Input: part model. Units: mm. Frame: model coordinates. Face numbers are marked on the shaded views. Coordinates: 2 decimals unless noted, no trailing zeros. Write each loop counter-clockwise with the first axis right and the second up, starting at its lowest first coordinate (ties: lowest second). Pieces come first, ordered by that corner, then holes. Notation, with made-up numbers: M 56,62 L 92,62 A31 cw 92,92 Z; hole C 26,50.5 d11. An arc over 180 degrees is marked long. Use CSV: the item, a comma, the result in double quotes.
```python
from build123d import *

# Parameters (mm, degrees)
SKETCH1_R           = 5.1
BOSS_EXTRUDE1_DEPTH = 4
BOSS_EXTRUDE2_START = -4
BOSS_EXTRUDE2_DEPTH = 4
SKETCH3_R           = 2.5
BOSS_EXTRUDE3_DEPTH = 4
SKETCH4_R           = 1.15
CUT_EXTRUDE1_DEPTH  = 4
FILLET1_R           = 10
FILLET2_R           = 1.5
FILLET3_R           = 5
SKETCH5_W           = 20.86
SKETCH5_H           = 29
BOSS_EXTRUDE4_DEPTH = 4
SKETCH6_W           = 4
SKETCH6_H           = 29
BOSS_EXTRUDE5_DEPTH = 12
FILLET4_R           = 10
FILLET5_R           = 2


with BuildPart() as part:
    # Sketch1 → Boss-Extrude1 (new body)
    with BuildSketch(Plane(origin=(0, 0, 0), x_dir=(1, 0, 0), z_dir=(0, 1, 0))):
        with BuildLine():
            ThreePointArc((-42.589636172, 29.834927363), (-52, 0), (-42.589636172, -29.834927363))
            ThreePointArc((-42.589636172, -29.834927363), (-41.790010768, -41.790010768), (-29.834927363, -42.589636172))
            ThreePointArc((-29.834927363, -42.589636172), (0, -52), (29.834927363, -42.589636172))
            ThreePointArc((29.834927363, -42.589636172), (41.790010768, -41.790010768), (42.589636172, -29.834927363))
            ThreePointArc((42.589636172, -29.834927363), (52, 0), (42.589636172, 29.834927363))
            ThreePointArc((42.589636172, 29.834927363), (41.790010768, 41.790010768), (29.834927363, 42.589636172))
            ThreePointArc((29.834927363, 42.589636172), (0, 52), (-29.834927363, 42.589636172))
            ThreePointArc((-29.834927363, 42.589636172), (-41.790010768, 41.790010768), (-42.589636172, 29.834927363))
        make_face()
        with Locations(Location((-35.355339059, -35.355339059, 0), (0, 0, 270))):
            Circle(SKETCH1_R, mode=Mode.SUBTRACT)
        with Locations(Location((35.355339059, -35.355339059, 0), (0, 0, 270))):
            Circle(SKETCH1_R, mode=Mode.SUBTRACT)
        with BuildLine():
            ThreePointArc((-27.258640426, -39.509068859), (-28.920667351, -28.920667351), (-39.509068859, -27.258640426))
            ThreePointArc((-39.509068859, -27.258640426), (-48, 0), (-39.509068859, 27.258640426))
            ThreePointArc((-39.509068859, 27.258640426), (-28.920667351, 28.920667351), (-27.258640426, 39.509068859))
            ThreePointArc((-27.258640426, 39.509068859), (0, 48), (27.258640426, 39.509068859))
            ThreePointArc((27.258640426, 39.509068859), (28.920667351, 28.920667351), (39.509068859, 27.258640426))
            ThreePointArc((39.509068859, 27.258640426), (48, 0), (39.509068859, -27.258640426))
            ThreePointArc((39.509068859, -27.258640426), (28.920667351, -28.920667351), (27.258640426, -39.509068859))
            ThreePointArc((27.258640426, -39.509068859), (0, -48), (-27.258640426, -39.509068859))
        make_face(mode=Mode.SUBTRACT)
        with Locations(Location((-35.355339059, 35.355339059, 0), (0, 0, 270))):
            Circle(SKETCH1_R, mode=Mode.SUBTRACT)
        with Locations(Location((35.355339059, 35.355339059, 0), (0, 0, 270))):
            Circle(SKETCH1_R, mode=Mode.SUBTRACT)
    extrude(amount=BOSS_EXTRUDE1_DEPTH)

    # Sketch2 → Boss-Extrude2 (add)
    with BuildSketch(Plane(origin=(0, 4, 0), x_dir=(1, 0, 0), z_dir=(0, 1, 0)).offset(BOSS_EXTRUDE2_START)):
        with BuildLine():
            ThreePointArc((-26.255339059, 35.355339059), (-26.311135203, 34.349169788), (-26.477839411, 33.355339059))
            Line((-26.477839411, 33.355339059), (26.477839411, 33.355339059))
            ThreePointArc((26.477839411, 33.355339059), (26.255339059, 35.355339059), (26.477839411, 37.355339059))
            Line((26.477839411, 37.355339059), (-26.477839411, 37.355339059))
            ThreePointArc((-26.477839411, 37.355339059), (-26.311135203, 36.36150833), (-26.255339059, 35.355339059))
        make_face()
        with BuildLine():
            Line((-33.355339059, -26.477839411), (-33.355339059, 26.477839411))
            ThreePointArc((-33.355339059, 26.477839411), (-35.355339059, 26.255339059), (-37.355339059, 26.477839411))
            Line((-37.355339059, 26.477839411), (-37.355339059, -26.477839411))
            ThreePointArc((-37.355339059, -26.477839411), (-35.355339059, -26.255339059), (-33.355339059, -26.477839411))
        make_face()
        with BuildLine():
            ThreePointArc((37.355339059, 26.477839411), (35.355339059, 26.255339059), (33.355339059, 26.477839411))
            Line((33.355339059, 26.477839411), (33.355339059, -26.477839411))
            ThreePointArc((33.355339059, -26.477839411), (35.355339059, -26.255339059), (37.355339059, -26.477839411))
            Line((37.355339059, -26.477839411), (37.355339059, 26.477839411))
        make_face()
        with BuildLine():
            Line((26.477839411, -33.355339059), (-26.477839411, -33.355339059))
            ThreePointArc((-26.477839411, -33.355339059), (-26.311135203, -34.349169788), (-26.255339059, -35.355339059))
            ThreePointArc((-26.255339059, -35.355339059), (-26.311135203, -36.36150833), (-26.477839411, -37.355339059))
            Line((-26.477839411, -37.355339059), (26.477839411, -37.355339059))
            ThreePointArc((26.477839411, -37.355339059), (26.255339059, -35.355339059), (26.477839411, -33.355339059))
        make_face()
    extrude(amount=BOSS_EXTRUDE2_DEPTH)

    # Sketch3 → Boss-Extrude3 (add)
    with BuildSketch(Plane(origin=(0, 4, 0), x_dir=(1, 0, 0), z_dir=(0, 1, 0))):
        with Locations((-20, 35.355339059)):
            Circle(SKETCH3_R)
        with Locations((20, 35.355339059)):
            Circle(SKETCH3_R)
        with Locations((35.355339059, 20)):
            Circle(SKETCH3_R)
        with Locations((35.355339059, -20)):
            Circle(SKETCH3_R)
        with Locations((-35.355339059, -20)):
            Circle(SKETCH3_R)
        with Locations((-35.355339059, 20)):
            Circle(SKETCH3_R)
        with Locations((-20, -35.355339059)):
            Circle(SKETCH3_R)
        with Locations((20, -35.355339059)):
            Circle(SKETCH3_R)
    extrude(amount=-BOSS_EXTRUDE3_DEPTH)

    # Sketch4 → Cut-Extrude1 (cut)
    with BuildSketch(Plane(origin=(0, 4, 0), x_dir=(1, 0, 0), z_dir=(0, 1, 0))):
        with Locations(Location((-20, 35.355339059, 0), (0, 0, 270))):
            Circle(SKETCH4_R)
        with Locations(Location((20, 35.355339059, 0), (0, 0, 270))):
            Circle(SKETCH4_R)
        with Locations(Location((-35.355339059, 20, 0), (0, 0, 270))):
            Circle(SKETCH4_R)
        with Locations(Location((-35.355339059, -20, 0), (0, 0, 270))):
            Circle(SKETCH4_R)
        with Locations(Location((-20, -35.355339059, 0), (0, 0, 270))):
            Circle(SKETCH4_R)
        with Locations(Location((20, -35.355339059, 0), (0, 0, 270))):
            Circle(SKETCH4_R)
        with Locations(Location((35.355339059, -20, 0), (0, 0, 270))):
            Circle(SKETCH4_R)
        with Locations(Location((35.355339059, 20, 0), (0, 0, 270))):
            Circle(SKETCH4_R)
    extrude(amount=-CUT_EXTRUDE1_DEPTH, mode=Mode.SUBTRACT)

    # Fillet1
    fillet1_edges = [part.edges().sort_by_distance(p)[0] for p in [
        (-42.589636172, 2, 29.834927363),
        (-42.589636172, 2, -29.834927363),
        (-29.834927363, 2, -42.589636172),
        (29.834927363, 2, -42.589636172),
        (42.589636172, 2, -29.834927363),
        (42.589636172, 2, 29.834927363),
        (29.834927363, 2, 42.589636172),
        (-29.834927363, 2, 42.589636172),
    ]]
    fillet(fillet1_edges, radius=FILLET1_R)

    # Fillet2
    fillet2_edges = [part.edges().sort_by_distance(p)[0] for p in [
        (37.355339059, 2, -26.477839411),
        (37.355339059, 2, 26.477839411),
        (-26.477839411, 2, 37.355339059),
        (26.477839411, 2, 37.355339059),
        (27.258640426, 2, 39.509068859),
        (39.509068859, 2, 27.258640426),
        (39.509068859, 2, -27.258640426),
        (27.258640426, 2, -39.509068859),
        (-27.258640426, 2, -39.509068859),
        (-39.509068859, 2, -27.258640426),
        (-39.509068859, 2, 27.258640426),
        (-27.258640426, 2, 39.509068859),
        (-26.477839411, 2, -37.355339059),
        (26.477839411, 2, -37.355339059),
        (-37.355339059, 2, -26.477839411),
        (-37.355339059, 2, 26.477839411),
    ]]
    fillet(fillet2_edges, radius=FILLET2_R)

    # Fillet3
    fillet3_edges = [part.edges().sort_by_distance(p)[0] for p in [
        (33.355339059, 2, -26.477839411),
        (33.355339059, 2, 26.477839411),
        (-26.477839411, 2, 33.355339059),
        (26.477839411, 2, 33.355339059),
        (-26.477839411, 2, -33.355339059),
        (26.477839411, 2, -33.355339059),
        (-33.355339059, 2, -26.477839411),
        (-33.355339059, 2, 26.477839411),
    ]]
    fillet(fillet3_edges, radius=FILLET3_R)

    # Sketch5 → Boss-Extrude4 (add)
    with BuildSketch(Plane(origin=(0, 4, 0), x_dir=(1, 0, 0), z_dir=(0, 1, 0))):
        with Locations((22.925339059, 0)):
            Rectangle(SKETCH5_W, SKETCH5_H)
    extrude(amount=-BOSS_EXTRUDE4_DEPTH)

    # Sketch6 → Boss-Extrude5 (add)
    with BuildSketch(Plane.XZ):
        with Locations((14.495339059, 0)):
            Rectangle(SKETCH6_W, SKETCH6_H)
    extrude(amount=BOSS_EXTRUDE5_DEPTH)

    # Fillet4
    # the kernel refuses this fillet: 10 mm, written as the material it takes off along each edge
    with BuildSketch(Plane(origin=(16.495339059, 0, -14.5), x_dir=(-1, 0, 0), z_dir=(0, -1, 0))) as fillet4_piece_1:
        with BuildLine():
            CenterArc((10, -8), FILLET4_R, 126.869897646, 53.130102354)
            Line((0, -8), (0, 0))
            Line((0, 0), (4, 0))
        make_face()
    extrude(amount=32, mode=Mode.SUBTRACT)
    with BuildSketch(Plane(origin=(16.495339059, 0, 14.5), x_dir=(0, 0, -1), z_dir=(0, -1, 0))) as fillet4_piece_2:
        with BuildLine():
            CenterArc((8, -10), FILLET4_R, 90, 53.130102354)
            Line((0, -4), (0, 0))
            Line((0, 0), (8, 0))
        make_face()
    extrude(amount=32, mode=Mode.SUBTRACT)

    # Fillet5
    fillet5_edges = [part.edges().sort_by_distance(p)[0] for p in [
        (33.355339059, 0, 16.5),
        (33.355339059, 2, -14.5),
        (33.355339059, 2, 14.5),
        (22.925339059, 0, -14.5),
        (22.925339059, 0, 14.5),
        (33.355339059, 0, -16.5),
    ]]
    fillet(fillet5_edges, radius=FILLET5_R)


solid = part.part
```
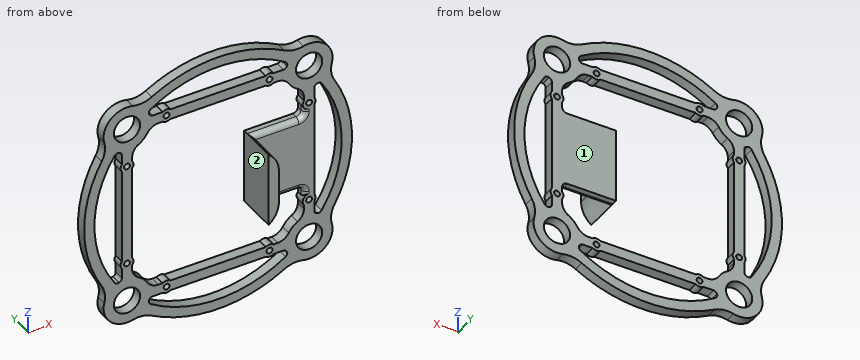
1. Material intervals for line 1 (X direction, y = 0.25, z = -37); line 2 (Z direction, x = -18, y = 2); line 3 (Z direction, x = -29.5, y = 2.75), sorted ascending. Write a range as [from, to].
Resolved:
line 1,"x = [-44.31, -40.18], [-30.53, 30.53], [40.18, 44.31]"
line 2,"z = [-48.79, -44.5], [-37.36, -33.36], [33.36, 37.36], [44.5, 48.79]"
line 3,"z = [-43.95, -28.39], [28.39, 43.95]"
2. Mould query, pull axis X, two halves, no side actions, for the marked faces 1 and 2. Classes: pulls with the +X half, pulls with the -X half, needs draft (parallel to the pull), parting line crosses it, or undercut.
Resolved:
face 1,"needs draft"
face 2,"undercut"
3. Section A-A (x = -9.5). Return loops of the section in (y, z), then the cut area to 3 significant figures.
Resolved:
outline,"M 0,-51.12 L 4,-51.12 L 4,-47.05 L 0,-47.05 Z; M 0,-37.36 L 4,-37.36 L 4,-33.36 L 0,-33.36 Z; M 0,33.36 L 4,33.36 L 4,37.36 L 0,37.36 Z; M 0,47.05 L 4,47.05 L 4,51.12 L 0,51.12 Z"
area,"64.6 mm^2"
4. Contact query for flat-ended pins moving along their axis: pin 1 Ø1.5 at (y, z) = (0, 41) entering from +X; pin 2 Ø0.6 at (y, z) = (3.5, 17.5) entering from -X; pin 3 Ø1.5 at (x, y) = (30.5, 1) entering from +Z; pin 4 Ø1.4 at (x, z) = (20, -35.36) entering from +Y. Output: stop coordinate, or through.
Resolved:
pin 1,"stops at x = 43.03"
pin 2,"stops at x = -49.07"
pin 3,"stops at z = 43.92"
pin 4,"passes through"
